Autodesk Inventor part; units mm, degrees
ref_plane "YZ Plane" through (0, 0, 0) normal (1, 0, 0) x (0, 1, 0)
ref_plane "XZ Plane" through (0, 0, 0) normal (0, 1, 0) x (-1, 0, 0)
ref_plane "XY Plane" through (0, 0, 0) normal (0, 0, 1) x (1, 0, 0)
sketch "Sketch1" plane through (0, 0, 0) normal (0, 0, 1) x (1, 0, 0)
  circle A0 centre (0, 0) radius 2
  arc A1 (-12.2474, 12.5) -> (12.2474, 12.5) centre (0, 0) ccw
  line L0 (-12.2474, 12.5) -> (12.2474, 12.5)
  dimension "d0" = 4
  dimension "d1" = 35
  dimension "d2" = 12.5
extrude "Extrusion1" add sketch "Sketch1" along normal blind 14
sketch "Sketch2" plane through (-12.2474, 12.5, 0) normal (0, 1, 0) x (1, 0, 0)
  line L0 (0, 0) -> (0, -14) construction
  line L1 (0, -7) -> (24.4949, -7) construction
  line L2 (24.4949, 0) -> (24.4949, -14) construction
  point P0 (12.2474, 0)
  point P1 (12.2474, -7)
hole "Hole1" at (0, 12.5, 7) direction (0, -1, 0) diameter 6.2 depth 12.5
sketch "Sketch4" plane through (0, 0, 14) normal (0, 0, 1) x (1, 0, 0)
  circle A0 centre (0, 0) radius 2
  circle A1 centre (0, 0) radius 2 construction
extrude "Extrusion3" add sketch "Sketch4" against normal blind 5
sketch "Sketch5" plane through (0, 0, 14) normal (0, 0, 1) x (1, 0, 0)
  point P0 (0, 0)
sketch "Sketch6" plane through (0, 0, 0) normal (0, 0, -1) x (-1, 0, 0)
  circle A0 centre (0, 0) radius 4
  circle A1 centre (0, 0) radius 5.5
  dimension "d16" = 8
  dimension "d29" = 1.5
extrude "Extrusion4" cut sketch "Sketch6" against normal blind 0.5
fillet "Fillet1" radius 0.5 2 edges at (4, 0, 0.5) (5.5, 0, 0.5)
fillet "Fillet2" radius 5 2 edges at (-12.2474, 12.5, 7) (12.2474, 12.5, 7)
sketch "Sketch8" plane through (0, 0, 14) normal (0, 0, 1) x (1, 0, 0)
  circle A0 centre (0, 0) radius 13 construction
  line L0 (-13, 0) -> (13, 0) construction
  line L1 (0, 0) -> (0, -13) construction
  dimension "d31" = 26
hole "Hole3" at (-13, 0, 14) at (13, 0, 14) at (0, -13, 14) direction (0, 0, -1) diameter 3.2 end through all counterbore diameter 5.8 counterbore depth 3
chamfer "Chamfer1" distance 1 angle 45 1 edges at (0, 12.5, 3.9)
properties part number "CH_01_0036_syringe_pump_mount" material "ABS Plastic"
The listing builds one solid part. Answer for the finished solid, in the listing's coordinates (mm). A direction names the side the tool comes from. Round coordinates to 2 decimals unless told otherwise and drop trailing zeros. Write each loop counter-clockwise with the first axis right and the second up, starting at its lowest first coordinate (ties: lowest second). Pieces come first, ordered by that corner, then holes. Notation, with made-up numbers: (-28.75, -34.5) -> (-4.75, -34.5) arc R36 cw to (-4.75, -0.5) -> close; hole circle Ø1 at (-8, 29.25). An arc over 180 degrees is marked (long way). Answer as a JSON object with one key per item and string values. Group by question number.
Q1. Each of these flat-tipped pins is pushed along its axis until it touches: pin 1 Ø8 at (x, z) = (0, 7) entering from +Y; pin 2 Ø5 at (y, z) = (8, 11.5) entering from -X; pin 3 Ø1.7 at (x, y) = (12.5, 1) entering from +Z. Where does it stop, or does it pass through?
Q2. Determine the mould class of faces 1 (the face through (0, 2, 9.4)), 2 (the face through (-12.207, 11.987, 7.098)), 3 (the face through (0, -6, 0)), 4 (the face through (-2.4, 0, 7)) for opening direction X: pulls with the +X half, pulls with the -X half, needs draft (parallel to the pull), parting line crosses it, or undercut.
Q3. Straight lines are drawn through the part: line 1 along X through (y, z) = (0, 2.5); line 2 along Y through (x, z) = (0, 7); line 3 along X through (y, z) = (0, 12.3). For each, find the intervals that lie inside material, in ascending order.
Q4. Section A-A (x = 0) is taken. Count the separate pieces of the cut face and the enclosed holes in it, plus the area to 3 significant figures.
Q5. Section D-D (y = 9) is taken. Write down the section's boundary in (x, z), plus the area to 3 significant figures.
Q6. Section B-B (z = 7) is taken. Write down the section's boundary in (x, y).
Q7. Which of the six approach directions +Z, -Z, +X, -X, +Y, -Y give full straight-line access (tool end or side, diameter ignored) to faces 5 (the face through (2.4, 0, 7)), 6 (the face through (0, -2, 3)), 7 (the face through (0, -2, 14)), 8 (the face through (-11.75, -1.25, 11))?
Q8. Section C-C (y = -13) is taken. Write down the section's boundary in (x, z), plus the area to 3 significant figures.
Check values:
{
 "1": {"pin 1": "y = 12.4", "pin 2": "x = -16.61", "pin 3": "z = 11"},
 "2": {"face 1": "undercut", "face 2": "pulls with the -X half", "face 3": "needs draft", "face 4": "undercut"},
 "3": {"line 1": "-17.5 to -14.6, -11.4 to -2, 2 to 11.4, 14.6 to 17.5", "line 2": "-17.5 to -14.6, -11.4 to -2", "line 3": "-17.5 to -15.9, -10.1 to 10.1, 15.9 to 17.5"},
 "4": {"separate pieces": "3", "enclosed holes": "0", "area": "264 mm^2"},
 "5": {"outline": "(-15.01, 0) -> (15.01, 0) -> (15.01, 14) -> (-15.01, 14) -> close; hole circle Ø6.2 at (0, 7)", "area": "390 mm^2"},
 "6": {"outline": "(-14, 10.5) arc R17.5 ccw (long way) to (14, 10.5) arc R5 ccw to (10, 12.5) -> (4.1, 12.5) -> (3.1, 11.5) -> (3.1, 0) -> (2, 0) arc R2 cw to (-2, 0) -> (-3.1, 0) -> (-3.1, 11.5) -> (-4.1, 12.5) -> (-10, 12.5) arc R5 ccw to start; hole circle Ø3.2 at (-13, 0); hole circle Ø3.2 at (0, -13); hole circle Ø3.2 at (13, 0)"},
 "7": {"face 5": "+Y", "face 6": "-Z", "face 7": "+Z, +X, -X, +Y, -Y", "face 8": "+Z"},
 "8": {"outline": "(-11.72, 0) -> (-1.6, 0) -> (-1.6, 11) -> (-2.9, 11) -> (-2.9, 14) -> (-11.72, 14) -> close; (1.6, 0) -> (11.72, 0) -> (11.72, 14) -> (2.9, 14) -> (2.9, 11) -> (1.6, 11) -> close", "area": "275 mm^2"}
}
